```python
from build123d import *

# Parameters (mm, degrees)
MAINBODY_EXTRUDE_START                 = -3
PROJECTIONXY_SKETCH_W                  = 20.5
PROJECTIONXY_SKETCH_H                  = 10
MAINBODY_EXTRUDE_DEPTH                 = 6
VISESCREWCLEARANCEHOLES_CUT_DEPTH      = 12.792476415
VISESCREWCLEARANCEHOLES_CUT_DEPTH_BACK = 12.792476415
VISESCREWCLEARANCEHOLES_SKETCH_R       = 2.625


with BuildPart() as part:
    # projectionXy_sketch → mainBody_extrude (new body)
    with BuildSketch(Plane.XY.offset(MAINBODY_EXTRUDE_START)):
        Rectangle(PROJECTIONXY_SKETCH_W, PROJECTIONXY_SKETCH_H)
    extrude(amount=MAINBODY_EXTRUDE_DEPTH)

    # viseScrewClearanceHoles_sketch → viseScrewClearanceHoles_cut (cut, two sides: drawn at the far end of the back side and taken through both)
    with BuildSketch(Plane.XY.offset(-VISESCREWCLEARANCEHOLES_CUT_DEPTH_BACK)):
        with Locations((-5.25, 0)):
            Circle(VISESCREWCLEARANCEHOLES_SKETCH_R)
        with Locations((5.25, 0)):
            Circle(VISESCREWCLEARANCEHOLES_SKETCH_R)
    extrude(amount=VISESCREWCLEARANCEHOLES_CUT_DEPTH + VISESCREWCLEARANCEHOLES_CUT_DEPTH_BACK, mode=Mode.SUBTRACT)


solid = part.part
```
Can you work these out from the model? Positions are in its coordinate system, mm. Coordinates: 2 decimals unless noted, no trailing zeros. Order: outer loops, then holes, each group sorted by start corner. A loop starts at its lowest first (then second) coordinate and runs counter-clockwise, first axis right, second up.
1. I'm going to push a flat-ended pin straight in: pin 1 (6 mm diameter, centred on x = 5.25, y = 0, fed in from +Z). Where does the tip first touch, or does it pass through?
2. If we section it at B-B (z = -1.5): Please give me the cut outline in (x, y) (3 decimals).
3. If we section it at A-A (x = -5.25): Please give me the cut outline in (y, z) (3 decimals), then the cut area to 3 significant figures.
4. If we section it at D-D (x = 6.5): Please give me the cut outline in (y, z), then the cut area to 3 significant figures.
5. I need wall thicknesses on line 1 (X direction, y = 0, z = -0.1) (3 decimals); line 2 (Y direction, x = -5.25, z = 1.6) (3 decimals); line 3 (X direction, y = 1.25, z = 1.4). Which ranges of each line are inside material? Lowest first, please.
6. Thinking about a two-plate mould opening in X: for faces 1 (the face through (-10.25, 0, 0)), 2 (the face through (0, 0, 3)), 3 (the face through (7.754, 0.788, -0.042)), 4 (the face through (-2.746, 0.788, -0.042)), which applies, +X half, -X half, draft (parallel to the pull), parting line (faces both ways), or undercut?
7. If we section it at C-C (y = 0.75): Please give me the cut outline in (x, z), then the cut area to 3 significant figures.
Entries:
1. pin 1: stops at z = 3
2. outline: (-10.25, -5) - (10.25, -5) - (10.25, 5) - (-10.25, 5) - close; hole circle Ø5.25 at (-5.25, 0); hole circle Ø5.25 at (5.25, 0)
3. outline: (-5, -3) - (-2.625, -3) - (-2.625, 3) - (-5, 3) - close; (2.625, -3) - (5, -3) - (5, 3) - (2.625, 3) - close
3. area: 28.5 mm2
4. outline: (-5, -3) - (-2.31, -3) - (-2.31, 3) - (-5, 3) - close; (2.31, -3) - (5, -3) - (5, 3) - (2.31, 3) - close
4. area: 32.3 mm2
5. line 1: x = -10.25 to -7.875, -2.625 to 2.625, 7.875 to 10.25
5. line 2: y = -5 to -2.625, 2.625 to 5
5. line 3: x = -10.25 to -7.56, -2.94 to 2.94, 7.56 to 10.25
6. face 1: -X half
6. face 2: draft
6. face 3: undercut
6. face 4: undercut
7. outline: (-10.25, -3) - (-7.77, -3) - (-7.77, 3) - (-10.25, 3) - close; (-2.73, -3) - (2.73, -3) - (2.73, 3) - (-2.73, 3) - close; (7.77, -3) - (10.25, -3) - (10.25, 3) - (7.77, 3) - close
7. area: 62.6 mm2
